from build123d import *

# Parameters (mm, degrees)
SKETCH1_R           = 17.5
SKETCH1_R_2         = 4
SKETCH1_R_3         = 1
BOSS_EXTRUDE1_DEPTH = 3.25
SKETCH2_R           = 1
CUT_EXTRUDE1_DEPTH  = 25.961219922


with BuildPart() as part:
    # Sketch1 → Boss-Extrude1 (new body)
    with BuildSketch(Plane.XY):
        with Locations(Location((0, 0, 0), (0, 0, 180))):
            Circle(SKETCH1_R)
        with Locations(Location((0, 0, 0), (0, 0, 180))):
            Circle(SKETCH1_R_2, mode=Mode.SUBTRACT)
        with Locations(Location((6.75, 0, 0), (0, 0, 180))):
            Circle(SKETCH1_R_3, mode=Mode.SUBTRACT)
        with Locations(Location((0, 8.75, 0), (0, 0, 180))):
            Circle(SKETCH1_R_3, mode=Mode.SUBTRACT)
        with Locations(Location((0, -8.75, 0), (0, 0, 180))):
            Circle(SKETCH1_R_3, mode=Mode.SUBTRACT)
        with Locations(Location((-6.75, 0, 0), (0, 0, 180))):
            Circle(SKETCH1_R_3, mode=Mode.SUBTRACT)
    extrude(amount=BOSS_EXTRUDE1_DEPTH)

    # Sketch2 → Cut-Extrude1 (cut, through all)
    with BuildSketch(Plane.XY.offset(3.25)):
        with Locations((11.522732664, -3.350616653)):
            Circle(SKETCH2_R)
        with Locations((-8.729040356, -8.530488981)):
            Circle(SKETCH2_R)
        with Locations((-3.08905487, 11.59799709)):
            Circle(SKETCH2_R)
    extrude(amount=-CUT_EXTRUDE1_DEPTH, mode=Mode.SUBTRACT)


solid = part.part
Verification items for the finished model (mm, model axes). Give positions to 0.01 mm unless a question says otherwise; leave off trailing zeros. Loops run counter-clockwise (first coordinate to the right, second up) from the corner with the lowest first, then second, coordinate; pieces in that order, holes last. Notation, with made-up numbers: (-27, 5.25) - (28, 5.25) arc R31 cw to (28, 35.25) - close; hole circle Ø5 at (-17, 41.5). An arc over 180 degrees is marked (long way). Write each question's results on one line, items separated by ' | '.
1) Sectioned sample at D-D on y = 8.75. Record the boundary of the cut face in (x, z).
Solution:
outline: (-15.16, 0) - (-1, 0) - (-1, 3.25) - (-15.16, 3.25) - close; (1, 0) - (15.16, 0) - (15.16, 3.25) - (1, 3.25) - close
2) Sectioned sample at B-B on x = 6.75. Record the boundary of the cut face in (y, z), plus the area to 3 significant figures.
Solution:
outline: (-16.15, 0) - (-1, 0) - (-1, 3.25) - (-16.15, 3.25) - close; (1, 0) - (16.15, 0) - (16.15, 3.25) - (1, 3.25) - close | area: 98.4 mm2
3) Sectioned sample at A-A on y = 0. Record the boundary of the cut face in (x, z), plus the area to 4 significant figures.
Solution:
outline: (-17.5, 0) - (-7.75, 0) - (-7.75, 3.25) - (-17.5, 3.25) - close; (-5.75, 0) - (-4, 0) - (-4, 3.25) - (-5.75, 3.25) - close; (4, 0) - (5.75, 0) - (5.75, 3.25) - (4, 3.25) - close; (7.75, 0) - (17.5, 0) - (17.5, 3.25) - (7.75, 3.25) - close | area: 74.75 mm2
4) Sectioned sample at C-C on z = 1.2. Count the separate pieces of the cut face and the enclosed holes in it, plus the area to 3 significant figures.
Solution:
separate pieces: 1 | enclosed holes: 8 | area: 890 mm2
5) Mould release check, pull along Y, two halves, no side actions. Record for faces 1 (the flat face through (-4, 4, 0)), 2 (the cylindrical face through (3.794, 17.084, 1.602)), 3 (the cylindrical face through (7.54, 0.61, 1.6)): pulls with the +Y half, pulls with the -Y half, needs draft (parallel to the pull), parting line crosses it, or undercut.
Solution:
face 1: needs draft | face 2: parting line crosses it | face 3: undercut
6) Depth check by flat-ended pin: P1, Ø1, axis at y = 2, z = 2.5, coming from the +X side; P2, Ø1, axis at y = 10, z = 2, coming from the +X side; P3, Ø1.5, axis at x = 7, z = 1, coming from the +Y side. Enter the tip coordinate at first touch or a pass-through.
Solution:
P1: x = 17.44 | P2: x = 14.7 | P3: y = 16.35
7) Material ranges on L1, parallel to Y at x = 0, z = 2.5; L2, parallel to X at y = -0.5, z = 2.55; L3, parallel to X at y = -2.5, z = 1.9, recorded low to high. Write a range as from..to.
Solution:
L1: -17.5..-9.75, -7.75..-4, 4..7.75, 9.75..17.5 | L2: -17.49..-7.62, -5.88..-3.97, 3.97..5.88, 7.62..17.49 | L3: -17.32..-3.12, 3.12..11, 12.05..17.32
